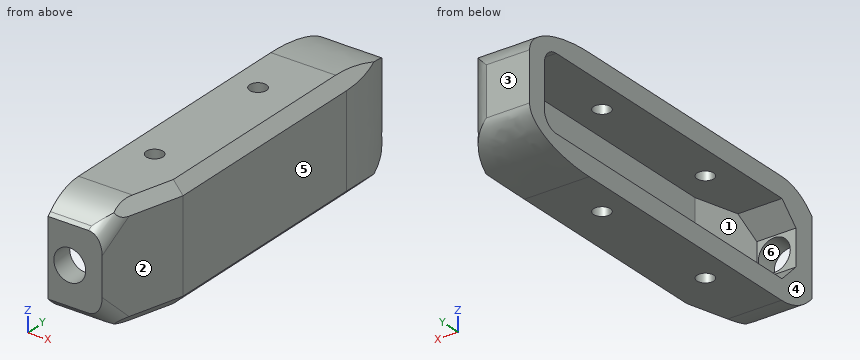
```python
from build123d import *

# Parameters (mm, degrees)
BOSS_EXTRU_1_DEPTH      = 21
COQUE1_START            = 3.7
COQUE1_DEPTH            = 13.6
ESQUISSE2_R             = 1.55
ENL_V_MAT_EXTRU_1_DEPTH = 32.5
ESQUISSE3_R             = 2.95
ENL_V_MAT_EXTRU_2_DEPTH = 10
CHANFREIN4_SIZE         = 3.5
CHANFREIN1_SIZE         = 2
CONG_1_R                = 3
CONG_2_DEPTH            = 11.330684872
CONG_3_SIZE             = 15
CONG_3_SIZE_2           = 6
CONG_4_SIZE             = 15
CONG_4_SIZE_2           = 6
CONG_5_SIZE             = 6
CONG_5_SIZE_2           = 15
CONG_6_R                = 3


with BuildPart() as part:
    # Esquisse1 → Boss.-Extru.1 (new body)
    with BuildSketch(Plane.XY):
        Polygon((0, 0), (10, 0), (14, 14.92820323), (14, 71.03), (0, 71.03), align=None)
    extrude(amount=BOSS_EXTRU_1_DEPTH)

    # Coque1: read off the stored shape, not the designer's step
    # Coque1 outline → Coque1 (cut)
    with BuildSketch(Plane.XY.offset(COQUE1_START)):
        Polygon((0, 4), (7.241274902, 4), (10.3, 15.415317471), (10.3, 67.33), (0, 67.33), align=None)
    extrude(amount=COQUE1_DEPTH, mode=Mode.SUBTRACT)

    # Esquisse2 → Enlèv. mat.-Extru.1 (cut)
    with BuildSketch(Plane.XY.offset(21)):
        with Locations((5, 46.03)):
            Circle(ESQUISSE2_R)
        with Locations((5, 20)):
            Circle(ESQUISSE2_R)
    extrude(amount=-ENL_V_MAT_EXTRU_1_DEPTH, mode=Mode.SUBTRACT)

    # Esquisse3 → Enlèv. mat.-Extru.2 (cut)
    with BuildSketch(Plane.XZ):
        with Locations(Location((4, 10.5, 0), (0, 0, 270))):
            Circle(ESQUISSE3_R)
    extrude(amount=-ENL_V_MAT_EXTRU_2_DEPTH, mode=Mode.SUBTRACT)

    # Chanfrein4
    chanfrein4_edges = [part.edges().sort_by_distance(p)[0] for p in [
        (3.620637451, 4, 3.7),
        (3.620637451, 4, 17.3),
        (5, 0, 0),
        (5, 0, 21),
    ]]
    chamfer(chanfrein4_edges, length=CHANFREIN4_SIZE)

    # Chanfrein1
    chanfrein1_edges = [part.edges().sort_by_distance(p)[0] for p in [
        (14, 42.979101615, 21),
        (14, 42.979101615, 0),
        (12.468911087, 9.214101615, 0),
        (12.468911087, 9.214101615, 21),
    ]]
    chamfer(chanfrein1_edges, length=CHANFREIN1_SIZE)

    # Congé1
    cong_1_edges = [part.edges().sort_by_distance(p)[0] for p in [
        (10.200961894, 0.75, 2.75),
        (10.200961894, 0.75, 18.25),
    ]]
    fillet(cong_1_edges, radius=CONG_1_R)

    # Congé2: read off the stored shape, not the designer's step
    # Congé2 outline → Congé2 (cut)
    with BuildSketch(Plane.YZ):
        with BuildLine():
            Line((3.5, 0), (7.642135624, 0))
            ThreePointArc((7.642135624, 0), (3.8153013, 0.761204675), (0.571067812, 2.928932188))
            Line((0.571067812, 2.928932188), (3.5, 0))
        make_face()
        with BuildLine():
            ThreePointArc((0.571067812, 18.071067812), (3.8153013, 20.238795325), (7.642135624, 21))
            Line((7.642135624, 21), (3.5, 21))
            Line((3.5, 21), (0.571067812, 18.071067812))
        make_face()
    extrude(amount=CONG_2_DEPTH, mode=Mode.SUBTRACT)

    # Congé3
    # a fillet whose section is not a circle: 15, 6 mm, written as the material it takes off along each edge
    with BuildSketch(Plane(origin=(49.5, 71.03, 21), x_dir=(0, -1, 0), z_dir=(-1, 0, 0))) as cong_3_piece_1:
        with BuildLine():
            Bezier((CONG_3_SIZE, 0), (0, 0), (0, -CONG_3_SIZE_2), weights=[1, 0.707106781, 1])
            Line((0, -CONG_3_SIZE_2), (0, 0))
            Line((0, 0), (CONG_3_SIZE, 0))
        make_face()
    extrude(amount=87, mode=Mode.SUBTRACT)

    # Congé4
    # a fillet whose section is not a circle: 15, 6 mm, written as the material it takes off along each edge
    with BuildSketch(Plane(origin=(49.5, 71.03, 0), x_dir=(0, -1, 0), z_dir=(-1, 0, 0))) as cong_4_piece_1:
        with BuildLine():
            Bezier((CONG_4_SIZE, 0), (0, 0), (0, CONG_4_SIZE_2), weights=[1, 0.707106781, 1])
            Line((0, CONG_4_SIZE_2), (0, 0))
            Line((0, 0), (CONG_4_SIZE, 0))
        make_face()
    extrude(amount=87, mode=Mode.SUBTRACT)

    # Congé5
    # a fillet whose section is not a circle: 15, 6 mm, written as the material it takes off along each edge
    with BuildSketch(Plane(origin=(14, 71.03, -31.5), x_dir=(-1, 0, 0), z_dir=(0, 0, 1))) as cong_5_piece_1:
        with BuildLine():
            Bezier((CONG_5_SIZE, 0), (0, 0), (0, CONG_5_SIZE_2), weights=[1, 0.707106781, 1])
            Line((0, CONG_5_SIZE_2), (0, 0))
            Line((0, 0), (CONG_5_SIZE, 0))
        make_face()
    extrude(amount=84, mode=Mode.SUBTRACT)

    # Congé6
    cong_6_edges = [part.edges().sort_by_distance(p)[0] for p in [
        (5.15, 67.33, 3.7),
        (5.15, 67.33, 17.3),
    ]]
    fillet(cong_6_edges, radius=CONG_6_R)


solid = part.part
```
Can you work these out from the model? Positions are in its coordinate system, mm. Face numbers are marked on the shaded views. A direction names the side the tool comes from. Coordinates: 2 decimals unless noted, no trailing zeros. Loops run counter-clockwise (first coordinate to the right, second up) from the corner with the lowest first, then second, coordinate; pieces in that order, holes last. Notation, with made-up numbers: (81, 75.25) -> (86, 75.25) arc R16 ccw to (86, 102.25) -> close; hole circle Ø8 at (28, 88.25). An arc over 180 degrees is marked (long way). Put each result on its own line as item: value. Start each with the question number.
Q1. For the marked faces 1 and 2, which set-ups out of +Z, -Z, +X, -X, +Y, -Y let a thin tool reach every point of the face, with its end or its side?
Q2. I want a section at A-A (y = 46.03). Write out the boundary of the cut face in (x, z), plus the area to 3 significant figures.
Q3. Thinking about a two-plate mould opening in X: for the marked faces 3, 4, 5 and 6, which applies, pulls with the +X half, pulls with the -X half, needs draft (parallel to the pull), parting line crosses it, or undercut?
Q4. If I drill on line 1 (Y direction, x = 5, z = 7.5); line 2 (Z direction, x = 1.25, y = 18); line 3 (Y direction, x = 5, z = 18.45), over which ranges is the centre line in solid material (lowest first)? Write a range as [from, to].
Q5. I want a section at B-B (y = 17.5). Write out the boundary of the cut face in (x, z).
Q6. I'm going to push flat-ended pins straight in: P1, Ø7, axis at y = 37, z = 13, coming from the -X side; P2, Ø1.5, axis at x = 12.5, y = 12, coming from the +Z side; P3, Ø1.9, axis at x = 5, y = 20, coming from the +Z side. Where does each tip first touch, or does it pass through?
Q7. I want a section at C-C (x = 5). Count the separate pieces of the cut face and the enclosed holes in it, plus the area to 3 significant figures.
Taken from the geometry:
1. face 1: -X
1. face 2: +Z, -Z, +X, -Y
2. outline: (0, 0) -> (3.45, 0) -> (3.45, 3.7) -> (0, 3.7) -> close; (0, 17.3) -> (3.45, 17.3) -> (3.45, 21) -> (0, 21) -> close; (6.55, 0) -> (12, 0) -> (14, 2) -> (14, 19) -> (12, 21) -> (6.55, 21) -> (6.55, 17.3) -> (10.3, 17.3) -> (10.3, 3.7) -> (6.55, 3.7) -> close
2. area: 127 mm2
3. face 3: needs draft
3. face 4: pulls with the -X half
3. face 5: pulls with the +X half
3. face 6: undercut
4. line 1: y = [0, 4], [67.33, 71.03]
4. line 2: z = [0, 3.7], [17.3, 21]
4. line 3: y = [0.97, 18.45], [21.55, 44.48], [47.58, 68.3]
5. outline: (0, 0) -> (12, 0) -> (14, 2) -> (14, 19) -> (12, 21) -> (0, 21) -> (0, 17.3) -> (10.3, 17.3) -> (10.3, 3.7) -> (0, 3.7) -> close
6. P1: stops at x = 10.3
6. P2: stops at z = 20.44
6. P3: passes through
7. separate pieces: 5
7. enclosed holes: 0
7. area: 523 mm2
